Check sheet for the modelled part. Datum: model origin and axes. Units: mm. A direction names the side the tool comes from. Coordinates: 2 decimals unless noted, no trailing zeros. Order: outer loops, then holes, each group sorted by start corner. A loop starts at its lowest first (then second) coordinate and runs counter-clockwise, first axis right, second up.
1. Cross-section at C-C (y = -26.5). Enter the section's corners in (x, z).
2. Draft check along X on faces 5 (the flat face through (2.54, -44, 36)), 6 (the flat face through (31, -86.36, 36)), 7 (the flat face through (52, -11, 35.56)). Enter one of: released by +X, released by -X, zero draft, split by the parting line, or undercut.
3. Thickness scan on line 1 (Y direction, x = 10.16, z = 32.8); line 2 (Y direction, x = 53.34, z = 34.05); line 3 (Y direction, x = 52, z = 33.5). Record the ranges inside material, lowest first.
4. Gauge pin test, flat ends, axial feed: pin 1 Ø14 at (x, y) = (14, -79.5) entering from +Z; pin 2 Ø4 at (x, y) = (55, -9.5) entering from +Z; pin 3 Ø3 at (x, z) = (32, 36.5) entering from -Y; pin 4 Ø8 at (x, y) = (44.5, -32) entering from +Z. Record the tip position at first contact, or that the pin passes through.
5. Set-up check for faces 1 (the cylindrical face through (3.989, -84.832, 36.222)), 2 (the cylindrical face through (59.511, -4.068, 36.222)), 3 (the flat face through (45.72, -78, 34)), 4 (the flat face through (17.78, -45, 23)): record each of +Z, -Z, +X, -X, +Y, -Y from which the full face is reachable in a straight line by a thin tool's end or side.
6. Cross-section at A-A (x = 26.5). Enter the section's corners in (y, z).
7. Cross-section at B-B (z = 22.5). Enter the section's corners in (x, y), then the cut area to 3 significant figures.
```python
from build123d import *

# Parameters (mm, degrees)
SKETCH1_W           = 63.5
SKETCH1_H           = 88.9
BOSS_EXTRUDE1_DEPTH = 38.1
SKETCH2_W           = 27.94
SKETCH2_H           = 50.8
CUT_EXTRUDE1_DEPTH  = 25.4
SKETCH3_W           = 53.34
SKETCH3_H           = 78.74
CUT_EXTRUDE2_DEPTH  = 5.08
SKETCH4_W           = 2.54
SKETCH4_H           = 12.7
BOSS_EXTRUDE2_DEPTH = 10.16
SKETCH5_W           = 12.7
SKETCH5_H           = 12.7
BOSS_EXTRUDE3_DEPTH = 2.54
SKETCH7_R           = 0.79375
CUT_EXTRUDE3_DEPTH  = 3.81
FILLET1_R           = 7.62
CUT_EXTRUDE4_DEPTH  = 3.81


with BuildPart() as part:
    # Sketch1 → Boss-Extrude1 (new body)
    with BuildSketch(Plane.XY):
        with Locations((31.75, -44.45)):
            Rectangle(SKETCH1_W, SKETCH1_H)
    extrude(amount=BOSS_EXTRUDE1_DEPTH)

    # Sketch2 → Cut-Extrude1 (cut)
    with BuildSketch(Plane.XY.offset(38.1)):
        with Locations((31.75, -44.45)):
            Rectangle(SKETCH2_W, SKETCH2_H)
    extrude(amount=-CUT_EXTRUDE1_DEPTH, mode=Mode.SUBTRACT)

    # Sketch3 → Cut-Extrude2 (cut)
    with BuildSketch(Plane.XY.offset(38.1)):
        with Locations((31.75, -44.45)):
            Rectangle(SKETCH3_W, SKETCH3_H)
    extrude(amount=-CUT_EXTRUDE2_DEPTH, mode=Mode.SUBTRACT)

    # Sketch4 → Boss-Extrude2 (add)
    with BuildSketch(Plane(origin=(17.78, 0, 0), x_dir=(0, 0, -1), z_dir=(1, 0, 0))):
        with Locations((-31.75, -45.007977767)):
            Rectangle(SKETCH4_W, SKETCH4_H)
    extrude(amount=BOSS_EXTRUDE2_DEPTH)

    # Sketch5 → Boss-Extrude3 (add)
    with BuildSketch(Plane.XY.offset(33.02)):
        with Locations((11.43, -11.43)):
            Rectangle(SKETCH5_W, SKETCH5_H)
        with Locations((52.07, -11.43)):
            Rectangle(SKETCH5_W, SKETCH5_H)
        with Locations((11.43, -77.47)):
            Rectangle(SKETCH5_W, SKETCH5_H)
        with Locations((52.07, -77.47)):
            Rectangle(SKETCH5_W, SKETCH5_H)
    extrude(amount=BOSS_EXTRUDE3_DEPTH)

    # Sketch7 → Cut-Extrude3 (cut)
    with BuildSketch(Plane.XY.offset(35.56)):
        with Locations((10.16, -11.43)):
            Circle(SKETCH7_R)
        with Locations((53.34, -11.43)):
            Circle(SKETCH7_R)
        with Locations((10.16, -77.449583408)):
            Circle(SKETCH7_R)
        with Locations((53.34, -77.449583408)):
            Circle(SKETCH7_R)
    extrude(amount=-CUT_EXTRUDE3_DEPTH, mode=Mode.SUBTRACT)

    # Fillet1
    fillet1_edges = [part.edges().sort_by_distance(p)[0] for p in [
        (0, 0, 19.05),
        (63.5, 0, 19.05),
        (63.5, -88.9, 19.05),
        (0, -88.9, 19.05),
    ]]
    fillet(fillet1_edges, radius=FILLET1_R)

    # Sketch8 → Cut-Extrude4 (cut)
    with BuildSketch(Plane.XY.offset(38.1)):
        with BuildLine():
            ThreePointArc((0, -81.28), (2.231846327, -86.668153673), (7.62, -88.9))
            Line((7.62, -88.9), (55.88, -88.9))
            ThreePointArc((55.88, -88.9), (61.268153673, -86.668153673), (63.5, -81.28))
            Line((63.5, -81.28), (63.5, -7.62))
            ThreePointArc((63.5, -7.62), (61.268153673, -2.231846327), (55.88, 0))
            Line((55.88, 0), (7.62, 0))
            ThreePointArc((7.62, 0), (2.231846327, -2.231846327), (0, -7.62))
            Line((0, -7.62), (0, -81.28))
        make_face()
        with BuildLine():
            ThreePointArc((7.62, -2.54), (3.984072808, -4.133699841), (2.54, -7.831604579))
            Line((2.54, -7.831604579), (2.54, -81.28))
            ThreePointArc((2.54, -81.28), (4.027897552, -84.872102448), (7.62, -86.36))
            Line((7.62, -86.36), (55.88, -86.36))
            ThreePointArc((55.88, -86.36), (59.472102448, -84.872102448), (60.96, -81.28))
            Line((60.96, -81.28), (60.96, -7.62))
            ThreePointArc((60.96, -7.62), (59.472102448, -4.027897552), (55.88, -2.54))
            Line((55.88, -2.54), (7.62, -2.54))
        make_face(mode=Mode.SUBTRACT)
    extrude(amount=-CUT_EXTRUDE4_DEPTH, mode=Mode.SUBTRACT)


solid = part.part
```
Data:
1. outline: (0, 0) - (63.5, 0) - (63.5, 34.29) - (60.96, 34.29) - (60.96, 38.1) - (58.42, 38.1) - (58.42, 33.02) - (45.72, 33.02) - (45.72, 12.7) - (17.78, 12.7) - (17.78, 33.02) - (5.08, 33.02) - (5.08, 38.1) - (2.54, 38.1) - (2.54, 34.29) - (0, 34.29) - close
2. face 5: released by -X
2. face 6: zero draft
2. face 7: undercut
3. line 1: y = -88.9 to -78.24, -76.66 to -12.22, -10.64 to 0
3. line 2: y = -88.9 to -78.24, -76.66 to -71.12, -17.78 to -12.22, -10.64 to 0
3. line 3: y = -88.9 to -71.12, -17.78 to 0
4. pin 1: stops at z = 38.1
4. pin 2: stops at z = 35.56
4. pin 3: stops at y = -86.36
4. pin 4: stops at z = 33.02
5. face 1: +Z, -X, -Y
5. face 2: +Z, +X, +Y
5. face 3: +Z
5. face 4: none
6. outline: (-88.9, 0) - (0, 0) - (0, 34.29) - (-2.54, 34.29) - (-2.54, 38.1) - (-5.08, 38.1) - (-5.08, 33.02) - (-19.05, 33.02) - (-19.05, 12.7) - (-69.85, 12.7) - (-69.85, 33.02) - (-83.82, 33.02) - (-83.82, 38.1) - (-86.36, 38.1) - (-86.36, 34.29) - (-88.9, 34.29) - close; (-51.36, 30.48) - (-38.66, 30.48) - (-38.66, 33.02) - (-51.36, 33.02) - close
7. outline: (0, -81.28) arc R7.62 ccw to (7.62, -88.9) - (55.88, -88.9) arc R7.62 ccw to (63.5, -81.28) - (63.5, -7.62) arc R7.62 ccw to (55.88, 0) - (7.62, 0) arc R7.62 ccw to (0, -7.62) - close; hole (17.78, -69.85) - (45.72, -69.85) - (45.72, -19.05) - (17.78, -19.05) - close
7. area: 4,180 mm2
